```python
from build123d import *

# Parameters (mm, degrees)
F1_DEPTH = 25


with BuildPart() as f1:
    # F0 (on Top) → F1 (new body)
    with BuildSketch(Plane.XY):
        with BuildLine():
            Line((-4.614562, 8.590986), (-9.337365, 8.590986))
            ThreePointArc((-9.337365, 8.590986), (-9.520423, 8.149044), (-9.962365, 7.965986))
            Line((-9.962365, 7.965986), (-9.962365, 7.518355))
            Line((-9.962365, 7.518355), (-9.952076, 7.091021))
            Line((-9.952076, 7.091021), (-3.989562, 7.091021))
            Line((-3.989562, 7.091021), (-3.989562, 7.965986))
            ThreePointArc((-3.989562, 7.965986), (-4.431504, 8.149044), (-4.614562, 8.590986))
        make_face()
        with BuildLine():
            ThreePointArc((-9.962365, 9.215986), (-9.520423, 9.032927), (-9.337365, 8.590986))
            Line((-9.337365, 8.590986), (-4.614562, 8.590986))
            ThreePointArc((-4.614562, 8.590986), (-4.431504, 9.032927), (-3.989562, 9.215986))
            Line((-3.989562, 9.215986), (-3.989562, 10.090986))
            Line((-3.989562, 10.090986), (-5.989562, 10.090986))
            Line((-5.989562, 10.090986), (-5.989562, 9.590986))
            Line((-5.989562, 9.590986), (-7.962365, 9.590986))
            Line((-7.962365, 9.590986), (-7.962365, 10.090986))
            Line((-7.962365, 10.090986), (-9.962365, 10.090986))
            Line((-9.962365, 10.090986), (-9.962365, 9.215986))
        make_face()
        with BuildLine():
            ThreePointArc((-9.962365, 7.965986), (-10.587365, 8.590986), (-9.962365, 9.215986))
            Line((-9.962365, 9.215986), (-9.962365, 10.090986))
            ThreePointArc((-9.962365, 10.090986), (-11.462356, 8.585842), (-9.952076, 7.091021))
            Line((-9.952076, 7.091021), (-9.962365, 7.518355))
            Line((-9.962365, 7.518355), (-9.962365, 7.965986))
        make_face()
        with BuildLine():
            Line((-3.989562, 10.090986), (-3.989562, 9.215986))
            ThreePointArc((-3.989562, 9.215986), (-3.547621, 9.032927), (-3.364562, 8.590986))
            ThreePointArc((-3.364562, 8.590986), (-3.547621, 8.149044), (-3.989562, 7.965986))
            Line((-3.989562, 7.965986), (-3.989562, 7.091021))
            ThreePointArc((-3.989562, 7.091021), (-2.48958, 8.591003), (-3.989562, 10.090986))
        make_face()
    extrude(amount=F1_DEPTH)


solid = f1.part
```
The listing builds one solid part. Answer for the finished solid, in the listing's coordinates (mm). Give positions to 0.01 mm unless a question says otherwise; leave off trailing zeros. Order: outer loops, then holes, each group sorted by start corner. A loop starts at its lowest first (then second) coordinate and runs counter-clockwise, first axis right, second up.
Item 1: The part is cut by section A-A, the plane x = -10.25. Give the vertices of the cut face in (y, z).
From the geometry:
outline: (7.12, 0) - (8.04, 0) - (8.04, 25) - (7.12, 25) - close; (9.15, 0) - (10.06, 0) - (10.06, 25) - (9.15, 25) - close
Item 2: The part is cut by section B-B, the plane z = 3. Give the vertices of the cut face in (x, y) (3 decimals), and give its area (3 significant figures).
From the geometry:
outline: (-9.962, 10.091) arc R1.5 ccw (long way) to (-9.952, 7.091) - (-3.99, 7.091) arc R1.5 ccw to (-3.99, 10.091) - (-5.99, 10.091) - (-5.99, 9.591) - (-7.962, 9.591) - (-7.962, 10.091) - close; hole circle Ø1.25 at (-9.962, 8.591); hole (-4.615, 8.591) arc R0.625 ccw to (-3.99, 7.966) arc R0.625 ccw to (-3.365, 8.591) arc R0.625 ccw to (-3.99, 9.216) arc R0.625 ccw to start
area: 21.5 mm2
Item 3: The part is cut by section D-D, the plane y = 7.45. Give the vertices of the cut face in (x, z).
From the geometry:
outline: (-10.94, 0) - (-3.02, 0) - (-3.02, 25) - (-10.94, 25) - close
Item 4: The part is cut by section C-C, the plane x = -6.25. Give the vertices of the cut face in (y, z), and give its area (3 significant figures).
From the geometry:
outline: (7.09, 0) - (9.59, 0) - (9.59, 25) - (7.09, 25) - close
area: 62.5 mm2
Item 5: For a pull along X with two mould halves and no side action, classify faces 1 (the face through (-7, 7.091, 12)), 2 (the face through (-7, 9.591, 12)), 3 (the face through (-2.49, 8.56, 12.32)) as pulls with the +X half, pulls with the -X half, needs draft (parallel to the pull), parting line crosses it, or undercut.
From the geometry:
face 1: needs draft
face 2: undercut
face 3: pulls with the +X half
Item 6: Find the intervals of material crossed by probe 1 along X at (y, z) = (8.5, 17.5); probe 2 along X at (y, z) = (8.25, 19); probe 3 along X at (y, z) = (9.7, 11.75), in increasing order.
From the geometry:
probe 1: x = -11.46 to -10.58, -9.34 to -4.61, -3.37 to -2.49
probe 2: x = -11.42 to -10.49, -9.44 to -4.51, -3.47 to -2.53
probe 3: x = -10.97 to -7.96, -5.99 to -2.98
